Design review of the part built by this model. Coordinates are the model's own, in mm. A direction names the side the tool comes from. Coordinates: 2 decimals unless noted, no trailing zeros. Loops run counter-clockwise (first coordinate to the right, second up) from the corner with the lowest first, then second, coordinate; pieces in that order, holes last. Notation, with made-up numbers: M 6.25,-17 L 11.25,-17 A6 ccw 11.25,-9 Z; hole C 76,4 d9. An arc over 180 degrees is marked long. One line per item, written item: value.
Autodesk Fusion 360 part; units mm, degrees
sketch "Sketch1" plane through (0, 0, 0) normal (0, 0, 1) x (1, 0, 0)
  circle A0 centre (0, 0) radius 3
  line L0 (15, -12.5) -> (-45, -12.5)
  line L1 (-45, -12.5) -> (-45, 12.5)
  line L2 (-45, 12.5) -> (15, 12.5)
  line L3 (15, 12.5) -> (15, -12.5)
  dimension "d1" = 6
  dimension "d2" = 25
  dimension "d12" = 60
  dimension "d14" = 15
extrude "Extrude1" add sketch "Sketch1" along normal blind 5
sketch "Sketch2" plane through (0, 0, 5) normal (0, 0, 1) x (-1, 0, 0)
  circle A0 centre (0, 0) radius 3
  line L0 (-15, -12.5) -> (45, -12.5)
  line L1 (45, -12.5) -> (45, 12.5)
  line L2 (45, 12.5) -> (-15, 12.5)
  line L3 (-15, 12.5) -> (-15, -12.5)
  line L4 (45, -12.5) -> (40, -12.5)
  line L5 (40, -12.5) -> (40, 12.5)
  line L6 (40, 12.5) -> (45, 12.5)
  line L7 (45, 12.5) -> (45, -12.5)
  dimension "d5" = 5
extrude "Extrude2" add sketch "Sketch2" along normal blind 40 contours L0 L1 L2 L4 L5 L6 L7
sketch "Sketch3" plane through (-40, 0, 0) normal (1, 0, 0) x (0, 1, 0)
  line L0 (-12.5, 5) -> (12.5, 5)
  line L1 (12.5, 5) -> (12.5, 45)
  line L2 (12.5, 45) -> (-12.5, 45)
  line L3 (-12.5, 45) -> (-12.5, 5)
  line L4 (6, 13.5) -> (-6, 13.5)
  line L5 (-6, 13.5) -> (-6, 36.5)
  line L6 (-6, 36.5) -> (6, 36.5)
  line L7 (6, 36.5) -> (6, 13.5)
  line L8 (6, 13.5) -> (-6, 36.5) construction
  line L9 (-6, 13.5) -> (6, 36.5) construction
  point P0 (0, 25)
  dimension "d8" = 12
  dimension "d9" = 23
extrude "Extrude3" cut sketch "Sketch3" against normal blind 40 contours L4 L5 L6 L7
(1) We need section C-C on y = 4. State the section outline as (x, z) points.
Reply:
outline: M -45,0 L 15,0 L 15,5 L -40,5 L -40,13.5 L -45,13.5 Z; M -45,36.5 L -40,36.5 L -40,45 L -45,45 Z
(2) To check wall thickness, follow line 1 along Y through (x, z) = (0, 4); line 2 along Z through (x, y) = (11.5, -0.5); line 3 along X through (y, z) = (9.5, 33). State the ranges of each line that lie inside material, in increasing order. Write a range as [from, to].
Reply:
line 1: y = [-12.5, -3], [3, 12.5]
line 2: z = [0, 5]
line 3: x = [-45, -40]
(3) Tool access review of faces 1 (the flat face through (-42, 0, 13.5)), 2 (the flat face through (-15, 0, 0)), 3 (the flat face through (-40, 9, 25)): name each direction out of +Z, -Z, +X, -X, +Y, -Y from which nothing blocks a thin tool from reaching the whole face with its end or side.
Reply:
face 1: +X, -X
face 2: -Z, +X, -X, +Y, -Y
face 3: +Z, +X, +Y, -Y
(4) Insertion check: pin 1 (3 mm diameter, centred on y = -3.5, z = 33.5, fed in from +X); pin 2 (6 mm diameter, centred on x = -3, y = 2.5, fed in from +Z); pin 3 (4 mm diameter, centred on y = -2.5, z = 36.5, fed in from +X); pin 4 (3 mm diameter, centred on x = -12.5, y = 1, fed in from -Z). Each pin has a flat end and moves straight along its axis. Give the tip position at first contact, or say it passes through.
Reply:
pin 1: passes through
pin 2: stops at z = 5
pin 3: stops at x = -40
pin 4: stops at z = 0
(5) Mouldability with a two-part tool opening along Z and no side actions: class faces 4 (the flat face through (-13, 0, 5)), 5 (the cylindrical face through (-3, 0, 2)), 6 (the flat face through (-42, -6, 25)), 7 (the flat face through (-42, 0, 36.5)) as released by +Z, released by -Z, zero draft, split by the parting line, or undercut.
Reply:
face 4: released by +Z
face 5: zero draft
face 6: undercut
face 7: undercut
(6) We need section A-A on y = 0. State the section outline as (x, z) points, then the cut area to 3 significant figures.
Reply:
outline: M -45,0 L -3,0 L -3,5 L -40,5 L -40,13.5 L -45,13.5 Z; M -45,36.5 L -40,36.5 L -40,45 L -45,45 Z; M 3,0 L 15,0 L 15,5 L 3,5 Z
area: 355 mm2
(7) We need section B-B on x = 0. State the section outline as (y, z) points, then the cut area to 3 significant figures.
Reply:
outline: M -12.5,0 L -3,0 L -3,5 L -12.5,5 Z; M 3,0 L 12.5,0 L 12.5,5 L 3,5 Z
area: 95.0 mm2
(8) We need section D-D on x = -41. State the section outline as (y, z) points.
Reply:
outline: M -12.5,0 L 12.5,0 L 12.5,45 L -12.5,45 Z; hole M -6,13.5 L 6,13.5 L 6,36.5 L -6,36.5 Z
